Here's how the part is built. I have some questions about the finished solid (model axes, mm). Face numbers are marked on the shaded views. A direction names the side the tool comes from. Round coordinates to 2 decimals unless told otherwise and drop trailing zeros. Loops run counter-clockwise (first coordinate to the right, second up) from the corner with the lowest first, then second, coordinate; pieces in that order, holes last. Notation, with made-up numbers: M 14.25,75 L 56.25,75 A11 cw 56.25,84 Z; hole C 79.25,-15 d2. An arc over 180 degrees is marked long. One line per question, with ' | ' between items. Start each with the question number.
Autodesk Inventor part; units mm, degrees
ref_plane "Płaszczyzna konstrukcyjna2" through (-49.4592, -8.3, 3) normal (0, 0, 1) x (1, 0, 0)
ref_plane "YZ Plane" through (0, 0, 0) normal (1, 0, 0) x (0, 1, 0)
ref_plane "XZ Plane" through (0, 0, 0) normal (0, 1, 0) x (-1, 0, 0)
ref_plane "Płaszczyzna konstrukcyjna1" through (0, 0, 0) normal (0, 0, 1) x (1, 0, 0)
sketch "Szkic1" plane through (0, 0, 0) normal (0, 0, 1) x (1, 0, 0)
  line L0 (-70.3592, -33) -> (-26.3592, -33)
  line L1 (-26.3592, -33) -> (-26.3592, -11)
  line L2 (-26.3592, -11) -> (-70.3592, -11)
  line L3 (-70.3592, -11) -> (-70.3592, -33)
  line L4 (-70.3592, -11) -> (-26.3592, -11)
  line L5 (-26.3592, -11) -> (-26.3592, -33)
  point P0 (0, 0)
extrude "Wyciągnięcie proste1" add sketch "Szkic1" against normal blind 3
sketch "Szkic2" plane through (0, 0, -3) normal (0, 0, -1) x (-1, 0, 0)
  line L0 (32.3592, -11) -> (26.3592, -11)
  line L1 (26.3592, -11) -> (26.3592, -33)
  line L2 (26.3592, -33) -> (32.3592, -33)
  line L3 (32.3592, -33) -> (32.3592, -11)
  line L4 (26.3592, -11) -> (26.3592, -33)
  line L5 (26.3592, -33) -> (70.3592, -33)
  line L6 (70.3592, -11) -> (26.3592, -11)
  point P0 (0, 0)
  dimension "d2" = 6
extrude "Wyciągnięcie proste2" add sketch "Szkic2" along normal blind 20
sketch "Szkic3" plane through (-26.3592, -33, 0) normal (1, 0, 0) x (0, 0, -1)
  circle A0 centre (6, 3.3) radius 1.25
  circle A1 centre (20, 3.3) radius 1.25
  circle A2 centre (20, 18.7) radius 1.25
  circle A3 centre (6, 18.7) radius 1.25
  circle A4 centre (20, 3.3) radius 1.5
  circle A5 centre (6, 3.3) radius 1.5
  circle A6 centre (20, 18.7) radius 1.5
  circle A7 centre (6, 18.7) radius 1.5
  circle A8 centre (13, 11) radius 2.125
  point P0 (0, 33)
  dimension "d5" = 0.25
  dimension "d6" = 0.25
  dimension "d7" = 0.25
  dimension "d8" = 0.25
extrude "Wyciągnięcie proste3" cut sketch "Szkic3" against normal through all contours A0 | A1 | A2 | A3 | A4 | A5 | A6 | A7 | A8
sketch "Szkic4" plane through (0, 0, 0) normal (0, 0, 1) x (1, 0, 0)
  line L0 (-40.9592, -22) -> (-40.9592, -11) construction
  line L1 (-70.3592, -11) -> (-32.3592, -11) construction
  line L2 (-40.9592, -22) -> (-40.9592, -33) construction
  line L3 (-70.3592, -33) -> (-26.3592, -33) construction
  line L4 (-26.3592, -33) -> (-26.3592, -11) construction
  line L5 (-55.5592, -11) -> (-26.3592, -11)
  line L6 (-26.3592, -11) -> (-26.3592, -33)
  line L7 (-26.3592, -33) -> (-55.5592, -33)
  line L8 (-55.5592, -33) -> (-55.5592, -11)
  line L9 (-40.9592, -22) -> (-55.5592, -22) construction
  line L10 (-40.9592, -22) -> (-26.3592, -22) construction
  line L11 (-26.3592, -11) -> (-70.3592, -11)
  point P0 (0, 0)
  dimension "d11" = 14.6
extrude "Wyciągnięcie proste4" cut sketch "Szkic4" against normal through all keep common part
ref_plane "Płaszczyzna konstrukcyjna2" through (-49.4592, -8.3, 3) normal (0, 0, 1) x (1, 0, 0)
sketch "Szkic5" plane through (0, 0, 0) normal (0, 0, 1) x (1, 0, 0)
  line L0 (-55.5592, -33) -> (-55.5592, -11)
  line L1 (-55.5592, -33) -> (-26.3592, -33)
  line L2 (-26.3592, -33) -> (-26.3592, -11)
  line L3 (-26.3592, -11) -> (-55.5592, -11)
  point P0 (0, 0)
extrude "Wyciągnięcie proste5" add sketch "Szkic5" along normal blind 3
hole "Otwór3" at (-40.9592, -22, 0) direction (0, 0, -1) diameter 4.25 end through all both
sketch "Szkic7" plane through (0, 0, 3) normal (0, 0, 1) x (1, 0, 0)
  circle A0 centre (-40.9592, -22) radius 10
  circle A1 centre (-40.9592, -22) radius 2.125
  circle A2 centre (-40.9592, -22) radius 10
  circle A3 centre (-40.9592, -22) radius 9.5
  point P0 (0, 0)
  dimension "d42" = 0.5
extrude "Wyciągnięcie proste8" add sketch "Szkic7" along normal blind 10 contours A3
sketch "Szkic6" plane through (0, 0, -3) normal (0, 0, -1) x (-1, 0, 0)
  circle A0 centre (40.9592, -22) radius 2.125
  circle A1 centre (40.9592, -22) radius 4.5
  point P0 (0, 0)
  dimension "d37" = 9
extrude "Wyciągnięcie proste7" cut sketch "Szkic6" against normal blind 12 contours A0 | A1
sketch "Szkic8" plane through (0, 0, -23) normal (0, 0, -1) x (-1, 0, 0)
  line L0 (26.3592, -33) -> (32.3592, -33)
  line L1 (32.3592, -33) -> (32.3592, -11)
  line L2 (32.3592, -11) -> (26.3592, -11)
  line L3 (26.3592, -11) -> (26.3592, -33)
  point P0 (0, 0)
extrude "Wyciągnięcie proste9" add sketch "Szkic8" along normal blind 18
mirror "Odbij1" about plane through (-29.3592, -22, -41) normal (0, 0, -1)
sketch "Szkic9" plane through (-32.3592, -33, -3) normal (-1, 0, 0) x (0, 0, 1)
  circle A0 centre (-66, 11) radius 2.125
  circle A1 centre (-59, 18.7) radius 1.5
  circle A2 centre (-59, 3.3) radius 1.5
  circle A3 centre (-73, 18.7) radius 1.5
  circle A4 centre (-73, 3.3) radius 1.5
  circle A5 centre (-3, 3.3) radius 1.5
  circle A6 centre (-3, 18.7) radius 1.5
  circle A7 centre (-17, 3.3) radius 1.5
  circle A8 centre (-17, 18.7) radius 1.5
  circle A9 centre (-10, 11) radius 2.125
  line L0 (0, 22) -> (0, 0)
  line L1 (0, 22) -> (-76, 22)
  line L2 (-76, 22) -> (-76, 0)
  line L3 (0, 0) -> (-76, 0)
  circle A10 centre (-66, 11) radius 2.125
  circle A11 centre (-66, 11) radius 4.5
  circle A12 centre (-10, 11) radius 2.125
  circle A13 centre (-10, 11) radius 4.5
  point P0 (3, 33)
  dimension "d47" = 9
  dimension "d48" = 9
extrude "Wyciągnięcie proste10" add sketch "Szkic9" along normal up to surface (23.2 mm away) contours L0 L3 L2 L1
sketch "Szkic11" plane through (-55.5592, -33, 3) normal (-1, 0, 0) x (0, 0, 1)
  line L0 (-86, 15.5) -> (-67.5, 15.5)
  line L1 (-67.5, 15.5) -> (-67.5, 6.5)
  line L2 (-67.5, 6.5) -> (-86, 6.5)
  line L3 (-86, 6.5) -> (-86, 15.5)
  line L4 (-20.5, 15.5) -> (-2, 15.5)
  line L5 (-2, 15.5) -> (-2, 6.5)
  line L6 (-2, 6.5) -> (-20.5, 6.5)
  line L7 (-20.5, 6.5) -> (-20.5, 15.5)
  line L8 (0, 22) -> (0, 0)
  line L9 (-88, 22) -> (-88, 0)
  circle A0 centre (-72, 11) radius 4.5
  circle A1 centre (-16, 11) radius 4.5
  point P0 (-3, 33)
  dimension "d51" = 2
  dimension "d53" = 2
extrude "Wyciągnięcie proste11" cut sketch "Szkic11" against normal blind 19.1
equation "\"d53\" = d51"
properties part number "wheel-adapter-rear"
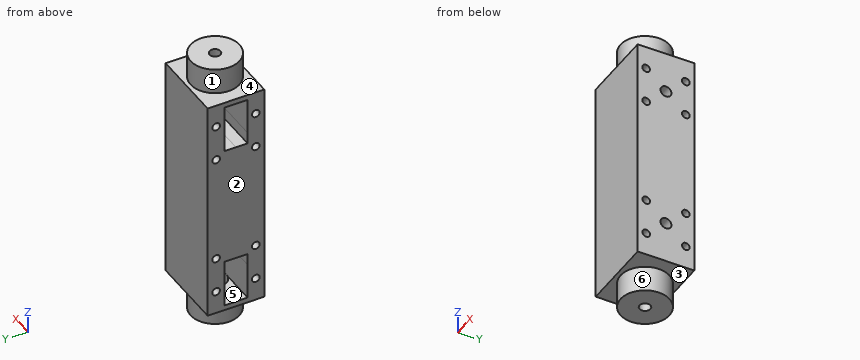
1) Imagine slicing it at A-A (z = -20). Write out the boundary of the cut face in (x, y), then the cut area to 3 significant figures.
2) Imagine slicing it at B-B (y = -29.7). Write out the boundary of the cut face in (x, z).
3) Imagine slicing it at C-C (x = -47.75). State how many separate pieces and enclosed holes the cut face has, then the cut area to 3 significant figures.
4) We'd pull the mould along Z, two halves only. Please class the marked faces 4, 5 and 6: pulls with the +Z half, pulls with the -Z half, needs draft (parallel to the pull), parting line crosses it, or undercut.
5) Imagine slicing it at D-D (z = 6). Write out the boundary of the cut face in (x, y), then the cut area to 3 significant figures.
6) For the marked faces 1, 2 and 3, which set-ups out of +Z, -Z, +X, -X, +Y, -Y let a thin tool reach every point of the face, with its end or its side?
7) Please list where these lines run through material, in increasing order: L1, parallel to Z at x = -40.25, y = -26; L2, parallel to Y at x = -37, z = -62; L3, parallel to Z at x = -42, y = -29.5. Write a range as from..to.
Results are:
1) outline: M -55.56,-33 L -26.36,-33 L -26.36,-31.2 L -55.56,-31.2 Z; M -55.56,-28.2 L -26.36,-28.2 L -26.36,-15.8 L -55.56,-15.8 Z; M -55.56,-12.8 L -26.36,-12.8 L -26.36,-11 L -55.56,-11 Z | area: 467 mm²
2) outline: M -55.56,-85 L -46.52,-85 L -46.52,-95 L -35.4,-95 L -35.4,-85 L -26.36,-85 L -26.36,-77.5 L -55.56,-77.5 Z; M -55.56,-74.5 L -26.36,-74.5 L -26.36,-63.5 L -55.56,-63.5 Z; M -55.56,-60.5 L -26.36,-60.5 L -26.36,-21.5 L -55.56,-21.5 Z; M -55.56,-18.5 L -26.36,-18.5 L -26.36,-7.5 L -55.56,-7.5 Z; M -55.56,-4.5 L -26.36,-4.5 L -26.36,3 L -35.4,3 L -35.4,13 L -46.52,13 L -46.52,3 L -55.56,3 Z
3) separate pieces: 1 | enclosed holes: 10 | area: 1,810 mm²
4) face 4: pulls with the +Z half | face 5: undercut | face 6: needs draft
5) outline: C -40.96,-22 d19; hole C -40.96,-22 d9 | area: 220 mm²
6) face 1: +Z | face 2: +Z, -Z, -X, +Y, -Y | face 3: -Z
7) L1: -95..-91, -64.5..-17.5, 9..13 | L2: -33..-31.2, -28.2..-15.8, -12.8..-11 | L3: -95..-77.49, -74.51..-63.49, -60.51..-21.49, -18.51..-7.49, -4.51..13
